Autodesk Inventor part; units mm, degrees
ref_plane "YZ Plane" through (0, 0, 0) normal (1, 0, 0) x (0, 1, 0)
ref_plane "XZ Plane" through (0, 0, 0) normal (0, 1, 0) x (-1, 0, 0)
ref_plane "XY Plane" through (0, 0, 0) normal (0, 0, 1) x (1, 0, 0)
ref_plane "Work Plane1" through (26.2088, 494.2322, 0) normal (0, 0, 1) x (-1, 0, 0)
sketch "Sketch1" plane through (26.2088, 494.2322, 0) normal (0, 0, 1) x (-1, 0, 0)
  line L0 (-27.8436, 404.4322) -> (-27.8436, 443.8322)
  line L1 (-27.8436, 404.4322) -> (-20.8436, 404.4322)
  line L2 (-20.8436, 404.4322) -> (-20.8436, 443.8322)
  line L3 (-27.8436, 443.8322) -> (-20.8436, 443.8322)
  arc A0 (-25.8436, 437.1322) -> (-21.8436, 437.1322) centre (-23.8436, 437.1322) ccw
  arc A1 (-21.8436, 437.1322) -> (-25.8436, 437.1322) centre (-23.8436, 437.1322) ccw
  arc A2 (-25.8436, 411.1322) -> (-21.8436, 411.1322) centre (-23.8436, 411.1322) ccw
  arc A3 (-21.8436, 411.1322) -> (-25.8436, 411.1322) centre (-23.8436, 411.1322) ccw
  line L4 (-52.8436, 404.4322) -> (-52.8436, 443.8322)
  line L5 (-52.8436, 404.4322) -> (-45.8436, 404.4322)
  line L6 (-45.8436, 404.4322) -> (-45.8436, 443.8322)
  line L7 (-52.8436, 443.8322) -> (-45.8436, 443.8322)
  arc A4 (-51.8436, 437.1322) -> (-47.8436, 437.1322) centre (-49.8436, 437.1322) ccw
  arc A5 (-47.8436, 437.1322) -> (-51.8436, 437.1322) centre (-49.8436, 437.1322) ccw
  arc A6 (-51.8436, 411.1322) -> (-47.8436, 411.1322) centre (-49.8436, 411.1322) ccw
  arc A7 (-47.8436, 411.1322) -> (-51.8436, 411.1322) centre (-49.8436, 411.1322) ccw
  line L8 (-45.8436, 520.2322) -> (-45.8436, 480.8322)
  line L9 (-45.8436, 520.2322) -> (-52.8436, 520.2322)
  line L10 (-52.8436, 520.2322) -> (-52.8436, 480.8322)
  line L11 (-45.8436, 480.8322) -> (-52.8436, 480.8322)
  arc A8 (-47.8436, 487.5322) -> (-51.8436, 487.5322) centre (-49.8436, 487.5322) ccw
  arc A9 (-51.8436, 487.5322) -> (-47.8436, 487.5322) centre (-49.8436, 487.5322) ccw
  arc A10 (-47.8436, 513.5322) -> (-51.8436, 513.5322) centre (-49.8436, 513.5322) ccw
  arc A11 (-51.8436, 513.5322) -> (-47.8436, 513.5322) centre (-49.8436, 513.5322) ccw
  line L12 (-20.8436, 520.2322) -> (-20.8436, 480.8322)
  line L13 (-20.8436, 520.2322) -> (-27.8436, 520.2322)
  line L14 (-27.8436, 520.2322) -> (-27.8436, 480.8322)
  line L15 (-20.8436, 480.8322) -> (-27.8436, 480.8322)
  arc A12 (-21.8436, 487.5322) -> (-25.8436, 487.5322) centre (-23.8436, 487.5322) ccw
  arc A13 (-25.8436, 487.5322) -> (-21.8436, 487.5322) centre (-23.8436, 487.5322) ccw
  arc A14 (-21.8436, 513.5322) -> (-25.8436, 513.5322) centre (-23.8436, 513.5322) ccw
  arc A15 (-25.8436, 513.5322) -> (-21.8436, 513.5322) centre (-23.8436, 513.5322) ccw
sketch "Sketch2" plane through (26.2088, 494.2322, 0) normal (0, 0, 1) x (-1, 0, 0)
  line L0 (-20.8436, 110.4465) -> (-27.8436, 110.4465)
  line L1 (10, 520.2322) -> (10, 480.8322)
  line L2 (-45.8436, 520.2322) -> (-52.8436, 520.2322)
  line L3 (-52.8436, 520.2322) -> (-52.8436, 480.8322)
  line L4 (-52.8436, 404.4322) -> (-45.8436, 404.4322)
  line L5 (-27.8436, 404.4322) -> (-20.8436, 404.4322)
  line L6 (-20.8436, 520.2322) -> (-52.8436, 520.2322)
  line L7 (-52.8436, 404.4322) -> (-20.8436, 404.4322)
  line L8 (159.1564, 465.2322) -> (159.1564, 375.2322)
  line L9 (124.1564, 453.4322) -> (67.7564, 453.4322) construction
  line L10 (67.7564, 453.4322) -> (67.7564, 397.0322) construction
  line L11 (67.7564, 397.0322) -> (124.1564, 397.0322) construction
  line L12 (124.1564, 397.0322) -> (124.1564, 453.4322) construction
  line L13 (159.1564, 375.2322) -> (94.1564, 375.2322)
  line L14 (94.1564, 375.2322) -> (-20.8436, 404.4322)
  line L15 (159.1564, 465.2322) -> (-20.8436, 520.2322)
  circle A0 centre (143.1564, 425.2322) radius 6.05
  circle A1 centre (48.7564, 425.2322) radius 6.05
  circle A2 centre (-23.8436, 513.5322) radius 2.25
  circle A3 centre (-23.8436, 487.5322) radius 2.25
  circle A4 centre (-23.8436, 437.1322) radius 2.25
  circle A5 centre (-23.8436, 411.1322) radius 2.25
  circle A6 centre (-49.8436, 411.1322) radius 2.25
  circle A7 centre (-49.8436, 437.1322) radius 2.25
  circle A8 centre (-49.8436, 487.5322) radius 2.25
  circle A9 centre (-49.8436, 513.5322) radius 2.25
  line L16 (-52.8436, 520.2322) -> (-56.8436, 520.2322)
  line L17 (-56.8436, 520.2322) -> (-56.8436, 404.4322)
  line L18 (-56.8436, 404.4322) -> (-52.8436, 404.4322)
  circle A10 centre (119.5264, 448.8022) radius 2.5
  circle A11 centre (119.5264, 401.6622) radius 2.5
  circle A12 centre (72.3864, 401.6622) radius 2.5
  circle A13 centre (72.3864, 448.8022) radius 2.5
  line L19 (119.5264, 448.8022) -> (119.5264, 401.6622) construction
  line L20 (119.5264, 401.6622) -> (72.3864, 401.6622) construction
  line L21 (119.5264, 448.8022) -> (72.3864, 401.6622) construction
  line L22 (119.5264, 401.6622) -> (72.3864, 448.8022) construction
  circle A14 centre (95.9564, 425.2322) radius 12
  circle A15 centre (143.1564, 442.7322) radius 2.75
  circle A16 centre (143.1564, 407.7322) radius 2.75
  circle A17 centre (48.7564, 407.7322) radius 2.75
  circle A18 centre (48.7564, 442.7322) radius 2.75
  circle A19 centre (110.8056, 410.383) radius 2.25
  circle A20 centre (110.8056, 440.0815) radius 2.25
  circle A21 centre (81.1071, 440.0815) radius 2.25
  circle A22 centre (81.1071, 410.383) radius 2.25
  arc A23 (-25.8436, 487.5322) -> (-21.8436, 487.5322) centre (-23.8436, 487.5322) ccw
  arc A24 (-25.8436, 513.5322) -> (-21.8436, 513.5322) centre (-23.8436, 513.5322) ccw
  line L23 (-53.8436, 520.2322) -> (-53.8436, 480.8322)
  line L24 (-56.8436, 520.2322) -> (-106.8436, 520.2322)
  line L25 (-106.8436, 520.2322) -> (-106.8436, 484.2322)
  line L26 (-106.8436, 484.2322) -> (-56.8436, 484.2322)
  circle A25 centre (-64.3436, 514.2322) radius 2.75
  circle A26 centre (-64.3436, 490.2322) radius 2.75
  circle A27 centre (-99.3436, 490.2322) radius 2.75
  circle A28 centre (-99.3436, 514.2322) radius 2.75
  line L27 (48.7564, 425.2322) -> (-81.8436, 425.2322) construction
  point P0 (26.2088, 494.2322)
  point P1 (-27.8436, 520.2322)
  point P2 (-20.8436, 480.8322)
  point P3 (124.1564, 425.2322)
  point P4 (159.1564, 420.2322)
  point P5 (-27.8436, 520.2322)
  point P6 (119.5264, 425.2322)
  point P7 (95.9564, 401.6622)
  point P8 (95.9564, 397.0322)
  point P9 (95.9564, 425.2322)
  dimension "d1" = 90
  dimension "d2" = 56.4
  dimension "d3" = 56.4
  dimension "d4" = 180
  dimension "d5" = 55
  dimension "d7" = 12.1
  dimension "d9" = 19
  dimension "d10" = 19
  dimension "d12" = 40
  dimension "d13" = 65
  dimension "d14" = 4.5
  dimension "d18" = 4
  dimension "d19" = 5
  dimension "d20" = 47.14
  dimension "d21" = 47.14
  dimension "d22" = 24
  dimension "d23" = 5.5
  dimension "d24" = 35
  dimension "d25" = 17.5
  dimension "d26" = 4.5
  dimension "d27" = 42
  dimension "d28" = 63.2
  dimension "d29" = 36
  dimension "d30" = 24
  dimension "d31" = 35
  dimension "d32" = 5.5
  dimension "d33" = 6
  dimension "d34" = 7.5
  dimension "d35" = 53
extrude "Extrusion1" add sketch "Sketch2" along normal blind 6
fillet "Fillet1" radius 8 6 edges at (-132.9476, 29, 3) (-132.9476, 119, 3) (-67.9476, 119, 3) (47.0524, -26, 3) (47.0524, 89.8, 3) (83.0524, 89.8, 3)
fillet "Fillet2" radius 2 3 edges at (133.0524, -26, 3) (133.0524, 10, 3) (83.0524, 10, 3)
equation "\"d10\" = d9"
equation "\"d25\" = 0.5 * d24"
properties part number "SIDE SUPPORT PLATES"
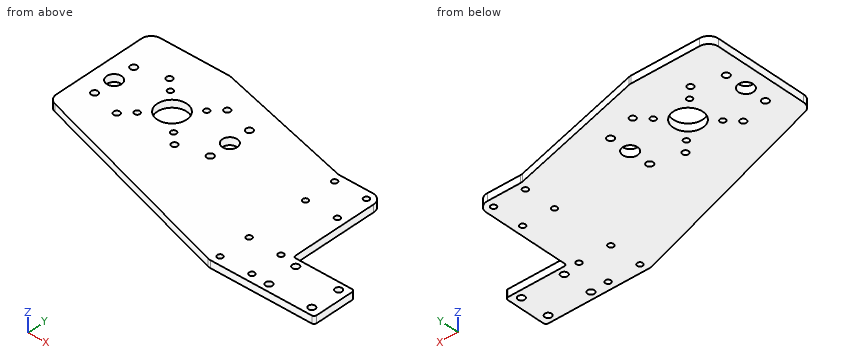
Build history of the part. All positions in model axes, mm. Coordinates: 2 decimals unless noted, no trailing zeros. Write each loop counter-clockwise with the first axis right and the second up, starting at its lowest first coordinate (ties: lowest second). Pieces come first, ordered by that corner, then holes.
(1) Cut at D-D on z = 0.95. State how many separate pieces and enclosed holes the cut face has, and give its area (3 significant figures).
(2) Cut at C-C on x = 108. List the corners of the cut face in (y, z), and give its area (3 significant figures).
(3) Drill centre lines: line 1 (X direction, y = 69, z = 3.25); line 2 (X direction, y = 59, z = 1.1); line 3 (Y direction, x = -24, z = 0.9). Where is each one in solid material? Low to high.
(4) Cut at B-B on y = 92.57. List the corners of the cut face in (x, z), and give its area (3 significant figures).
(5) Pin check, flat tips, straight feed: pin 1 Ø6 at (x, y) = (-54.9, 54.15) entering from +Z; pin 2 Ø2.5 at (x, y) = (50.05, -19.3) entering from +Z; pin 3 Ø3 at (x, z) = (7, 1.5) entering from +Y; pin 4 Ø1.5 at (y, z) = (58.5, 1) entering from +X. Stop position of each tip, or through.
(6) Cut at A-A on y = 69. List the corners of the cut face in (x, z), and give its area (3 significant figures).
Working result:
1. separate pieces: 1
1. enclosed holes: 27
1. area: 24,300 mm2
2. outline: (-26, 0) - (10, 0) - (10, 6) - (-26, 6) - close
2. area: 216 mm2
3. line 1: x = -132.95 to -123, -110.9 to -81.75, -57.75 to -28.6, -16.5 to 83.05
3. line 2: x = -132.95 to -76.38, -63.11 to 48.85, 51.26 to 74.85, 77.26 to 83.05
3. line 3: y = -4.29 to 49.16, 53.84 to 63.13, 74.87 to 84.16, 88.84 to 107.84
4. outline: (-132.95, 0) - (-95.82, 0) - (-95.82, 6) - (-132.95, 6) - close; (-90.82, 0) - (-48.68, 0) - (-48.68, 6) - (-90.82, 6) - close; (-43.68, 0) - (36.14, 0) - (36.14, 6) - (-43.68, 6) - close
4. area: 955 mm2
5. pin 1: stops at z = 6
5. pin 2: passes through
5. pin 3: stops at y = 100.35
5. pin 4: stops at x = 83.05
6. outline: (-132.95, 0) - (-123, 0) - (-123, 6) - (-132.95, 6) - close; (-110.9, 0) - (-81.75, 0) - (-81.75, 6) - (-110.9, 6) - close; (-57.75, 0) - (-28.6, 0) - (-28.6, 6) - (-57.75, 6) - close; (-16.5, 0) - (83.05, 0) - (83.05, 6) - (-16.5, 6) - close
6. area: 1,010 mm2
